from build123d import *

# Parameters (mm, degrees)
SKETCH1_R           = 5.55625
SKETCH1_R_2         = 31.75
SKETCH1_R_3         = 27.94
BOSS_EXTRUDE1_DEPTH = 6.35
SKETCH2_R           = 31.75
SKETCH2_R_2         = 27.94
BOSS_EXTRUDE2_DEPTH = 12.7


with BuildPart() as part:
    # Sketch1 → Boss-Extrude1 (new body)
    # profile 1 of 6: a face of its own
    with BuildSketch(Plane(origin=(0, 0, 0), x_dir=(1, 0, 0), z_dir=(0, 1, 0))):
        with BuildLine():
            ThreePointArc((-58.292365076, 0), (-62.236852489, 8.036977248), (-71.007523203, 9.833451426))
            ThreePointArc((-71.007523203, 9.833451426), (-78.611836011, 0.103683747), (-71.207683119, -9.7792547))
            Line((-71.207683119, -9.7792547), (-70.807129229, -9.883353974))
            ThreePointArc((-70.807129229, -9.883353974), (-62.155492987, -7.973393374), (-58.292365076, 0))
        make_face()
        with Locations(Location((-68.452365076, 0, 0), (0, 0, 270))):
            Circle(SKETCH1_R, mode=Mode.SUBTRACT)
    # profile 2 of 6: a face of its own
    with BuildSketch(Plane(origin=(0, 0, 0), x_dir=(1, 0, 0), z_dir=(0, 1, 0))):
        with BuildLine():
            Line((-9.883353974, 70.807129229), (-18.697333242, 36.892640474))
            ThreePointArc((-18.697333242, 36.892640474), (-25.320558446, 25.320679007), (-36.892798129, 18.697939919))
            Line((-36.892798129, 18.697939919), (-71.007523203, 9.833451426))
            ThreePointArc((-71.007523203, 9.833451426), (-62.236852489, 8.036977248), (-58.292365076, 0))
            ThreePointArc((-58.292365076, 0), (-62.155492987, -7.973393374), (-70.807129229, -9.883353974))
            Line((-70.807129229, -9.883353974), (-36.892640474, -18.697333242))
            ThreePointArc((-36.892640474, -18.697333242), (-25.320679007, -25.320558446), (-18.697939919, -36.892798129))
            Line((-18.697939919, -36.892798129), (-9.833451426, -71.007523203))
            ThreePointArc((-9.833451426, -71.007523203), (-1.287970014, -58.374332865), (10.16, -68.452365076))
            ThreePointArc((10.16, -68.452365076), (10.090601478, -69.637844646), (9.883353974, -70.807129229))
            Line((9.883353974, -70.807129229), (18.697333242, -36.892640474))
            ThreePointArc((18.697333242, -36.892640474), (25.320558446, -25.320679007), (36.892798129, -18.697939919))
            Line((36.892798129, -18.697939919), (71.007523203, -9.833451426))
            ThreePointArc((71.007523203, -9.833451426), (58.292889794, -0.103256972), (70.807129229, 9.883353974))
            Line((70.807129229, 9.883353974), (36.892640474, 18.697333242))
            ThreePointArc((36.892640474, 18.697333242), (25.320679007, 25.320558446), (18.697939919, 36.892798129))
            Line((18.697939919, 36.892798129), (9.833451426, 71.007523203))
            ThreePointArc((9.833451426, 71.007523203), (10.078032211, 69.74033509), (10.16, 68.452365076))
            ThreePointArc((10.16, 68.452365076), (-1.18547957, 58.361763598), (-9.883353974, 70.807129229))
        make_face()
        Circle(SKETCH1_R_2, mode=Mode.SUBTRACT)
    # profile 3 of 6: a face of its own
    with BuildSketch(Plane(origin=(0, 0, 0), x_dir=(1, 0, 0), z_dir=(0, 1, 0))):
        with BuildLine():
            ThreePointArc((10.16, -68.452365076), (-1.287970014, -58.374332865), (-9.833451426, -71.007523203))
            ThreePointArc((-9.833451426, -71.007523203), (-0.103683747, -78.611836011), (9.7792547, -71.207683119))
            Line((9.7792547, -71.207683119), (9.883353974, -70.807129229))
            ThreePointArc((9.883353974, -70.807129229), (10.090601478, -69.637844646), (10.16, -68.452365076))
        make_face()
        with Locations(Location((0, -68.452365076, 0), (0, 0, 270))):
            Circle(SKETCH1_R, mode=Mode.SUBTRACT)
    # profile 4 of 6: a face of its own
    with BuildSketch(Plane(origin=(0, 0, 0), x_dir=(1, 0, 0), z_dir=(0, 1, 0))):
        with BuildLine():
            Line((-9.7792547, 71.207683119), (-9.883353974, 70.807129229))
            ThreePointArc((-9.883353974, 70.807129229), (-1.18547957, 58.361763598), (10.16, 68.452365076))
            ThreePointArc((10.16, 68.452365076), (10.078032211, 69.74033509), (9.833451426, 71.007523203))
            ThreePointArc((9.833451426, 71.007523203), (0.103683747, 78.611836011), (-9.7792547, 71.207683119))
        make_face()
        with Locations(Location((0, 68.452365076, 0), (0, 0, 270))):
            Circle(SKETCH1_R, mode=Mode.SUBTRACT)
    # profile 5 of 6: a face of its own
    with BuildSketch(Plane(origin=(0, 0, 0), x_dir=(1, 0, 0), z_dir=(0, 1, 0))):
        with BuildLine():
            Line((71.207683119, 9.7792547), (70.807129229, 9.883353974))
            ThreePointArc((70.807129229, 9.883353974), (58.292889794, -0.103256972), (71.007523203, -9.833451426))
            ThreePointArc((71.007523203, -9.833451426), (76.489342324, -6.215512587), (78.612365076, 0))
            ThreePointArc((78.612365076, 0), (76.552353697, 6.133170823), (71.207683119, 9.7792547))
        make_face()
        with Locations(Location((68.452365076, 0, 0), (0, 0, 270))):
            Circle(SKETCH1_R, mode=Mode.SUBTRACT)
    # profile 6 of 6: a face of its own
    with BuildSketch(Plane(origin=(0, 0, 0), x_dir=(1, 0, 0), z_dir=(0, 1, 0))):
        Circle(SKETCH1_R_2)
        with Locations(Location((0, 0, 0), (0, 0, 270))):
            Circle(SKETCH1_R_3, mode=Mode.SUBTRACT)
    extrude(amount=BOSS_EXTRUDE1_DEPTH)

    # Sketch2 → Boss-Extrude2 (add)
    with BuildSketch(Plane(origin=(0, 6.35, 0), x_dir=(1, 0, 0), z_dir=(0, 1, 0))):
        with Locations(Location((0, 1.038430884, 0), (0, 0, 270))):
            Circle(SKETCH2_R)
        with Locations(Location((0, 0, 0), (0, 0, 270))):
            Circle(SKETCH2_R_2, mode=Mode.SUBTRACT)
    extrude(amount=BOSS_EXTRUDE2_DEPTH)


solid = part.part
CAD build for the part. Positions are in the model's coordinates, mm. A direction names the side the tool comes from. Give positions to 0.01 mm unless a question says otherwise; leave off trailing zeros. Order: outer loops, then holes, each group sorted by start corner. A loop starts at its lowest first (then second) coordinate and runs counter-clockwise, first axis right, second up. Notation, with made-up numbers: (33, 75) - (58, 75) arc R28 ccw to (58, 112) - close; hole circle Ø2 at (41, -37.75). An arc over 180 degrees is marked (long way). Write each question's results on one line, items separated by ' | '.
1. 3-axis set-ups, long thin cutter, end or side, ignore diameter. For faces 1 (the face through (-31, 12.6, -7.9)), 2 (the face through (14.33, 3.13, -53.71)): which of +Z, -Z, +X, -X, +Y, -Y reach the whole face in a straight line?
Calculated:
face 1: +Y | face 2: -Z, +X, +Y, -Y
2. Saw through at C-C on y = 4.5. List the corners of the cut face in (x, z), and give its area (3 significant figures).
Calculated:
outline: (-71.21, 9.78) arc R10.16 ccw to (-71.01, -9.83) - (-36.89, -18.7) arc R25.4 cw to (-18.7, -36.89) - (-9.78, -71.21) arc R10.16 ccw to (9.83, -71.01) - (18.7, -36.89) arc R25.4 cw to (36.89, -18.7) - (71.21, -9.78) arc R10.16 ccw to (71.01, 9.83) - (36.89, 18.7) arc R25.4 cw to (18.7, 36.89) - (9.78, 71.21) arc R10.16 ccw to (-9.83, 71.01) - (-18.7, 36.89) arc R25.4 cw to (-36.89, 18.7) - close; hole circle Ø11.11 at (-68.45, 0); hole circle Ø55.88 at (0, 0); hole circle Ø11.11 at (0, -68.45); hole circle Ø11.11 at (0, 68.45); hole circle Ø11.11 at (68.45, 0) | area: 6,030 mm2
3. Probe L1, parallel to X at y = 13.25, z = 0; L2, parallel to Z at x = -12, y = 12.75; L3, parallel to X at y = 4.25, z = 67. List the from-to ranges inside material, lowest first. Write a range as from..to.
Calculated:
L1: x = -31.73..-27.94, 27.94..31.73 | L2: z = -30.43..-25.23, 25.23..28.36 | L3: x = -10.87..-5.36, 5.36..10.87
4. Saw through at D-D on x = 21. List the corners of the cut face in (y, z), and give its area (3 significant figures).
Calculated:
outline: (0, -31.09) - (6.35, -31.09) - (6.35, -24.85) - (19.05, -24.85) - (19.05, -18.43) - (0, -18.43) - close; (0, 18.43) - (19.05, 18.43) - (19.05, 22.77) - (6.35, 22.77) - (6.35, 31.09) - (0, 31.09) - close | area: 297 mm2
5. Saw through at B-B on z = -12. List the corners of the cut face in (x, y), and give its area (3 significant figures).
Calculated:
outline: (-62.67, 0) - (-25.23, 0) - (-25.23, 19.05) - (-29.8, 19.05) - (-29.8, 6.35) - (-62.67, 6.35) - close; (25.23, 0) - (62.66, 0) - (62.66, 6.35) - (29.8, 6.35) - (29.8, 19.05) - (25.23, 19.05) - close | area: 591 mm2
6. Saw through at A-A on x = 0. List the corners of the cut face in (y, z), and give its area (3 significant figures).
Calculated:
outline: (0, -78.61) - (6.35, -78.61) - (6.35, -74.01) - (0, -74.01) - close; (0, -62.9) - (6.35, -62.9) - (6.35, -32.79) - (19.05, -32.79) - (19.05, -27.94) - (0, -27.94) - close; (0, 27.94) - (19.05, 27.94) - (19.05, 30.71) - (6.35, 30.71) - (6.35, 62.9) - (0, 62.9) - close; (0, 74.01) - (6.35, 74.01) - (6.35, 78.61) - (0, 78.61) - close | area: 599 mm2
7. Pin check, flat tips, straight feed: pin 1 (13 mm diameter, centred on x = -68.45, z = 0, fed in from +Y); pin 2 (1 mm diameter, centred on y = 12, z = 9, fed in from +X); pin 3 (5 mm diameter, centred on x = 24, y = 6.5, fed in from -Z). Stop position of each tip, or through.
Calculated:
pin 1: stops at y = 6.35 | pin 2: stops at x = 30.28 | pin 3: stops at z = -30.21
8. Pull direction X, two halves, no side cores. Call faces 3 (the face through (-25.19, 3.13, -25.45)), 4 (the face through (-73.876, 3.131, -1.204)), 5 (the face through (0.244, 3.131, -74.003)), 6 (the face through (0.29, 3.13, -78.61)): released by +X, released by -X, zero draft, split by the parting line, or undercut.
Calculated:
face 3: released by -X | face 4: undercut | face 5: undercut | face 6: split by the parting line
